from build123d import *

# Parameters (mm, degrees)
BOSS_EXTRUDE1_DEPTH = 120
SKETCH3_W           = 42
SKETCH3_H           = 12
CUT_EXTRUDE2_DEPTH  = 30
SKETCH6_R           = 2.5
CUT_EXTRUDE3_DEPTH  = 30
SKETCH8_W           = 42.8
SKETCH8_H           = 12.8
BOSS_EXTRUDE2_DEPTH = 30
SKETCH9_R           = 2.5
CUT_EXTRUDE4_DEPTH  = 30


with BuildPart() as part:
    # Sketch1 → Boss-Extrude1 (new body)
    with BuildSketch(Plane(origin=(0, 0, 0), x_dir=(1, 0, 0), z_dir=(0, 1, 0))):
        with BuildLine():
            Line((2, 0), (48, 0))
            ThreePointArc((48, 0), (49.414213562, 0.585786438), (50, 2))
            Line((50, 2), (50, 18))
            ThreePointArc((50, 18), (49.414213562, 19.414213562), (48, 20))
            Line((48, 20), (2, 20))
            ThreePointArc((2, 20), (0.585786438, 19.414213562), (0, 18))
            Line((0, 18), (0, 2))
            ThreePointArc((0, 2), (0.585786438, 0.585786438), (2, 0))
        make_face()
    extrude(amount=BOSS_EXTRUDE1_DEPTH)

    # Sketch3 → Cut-Extrude2 (cut)
    with BuildSketch(Plane.XZ):
        with Locations((25, -10)):
            Rectangle(SKETCH3_W, SKETCH3_H)
    extrude(amount=-CUT_EXTRUDE2_DEPTH, mode=Mode.SUBTRACT)

    # Sketch6 → Cut-Extrude3 (cut)
    with BuildSketch(Plane.XY):
        with Locations((25, 105)):
            Circle(SKETCH6_R)
        with Locations((25, 15)):
            Circle(SKETCH6_R)
    extrude(amount=-CUT_EXTRUDE3_DEPTH, mode=Mode.SUBTRACT)

    # Sketch8 → Boss-Extrude2 (add)
    with BuildSketch(Plane(origin=(0, 120, 0), x_dir=(1, 0, 0), z_dir=(0, 1, 0))):
        with Locations((25, 10)):
            Rectangle(SKETCH8_W, SKETCH8_H)
    extrude(amount=BOSS_EXTRUDE2_DEPTH)

    # Sketch9 → Cut-Extrude4 (cut)
    with BuildSketch(Plane.XY.offset(-3.6)):
        with Locations((25, 135)):
            Circle(SKETCH9_R)
    extrude(amount=-CUT_EXTRUDE4_DEPTH, mode=Mode.SUBTRACT)


solid = part.part
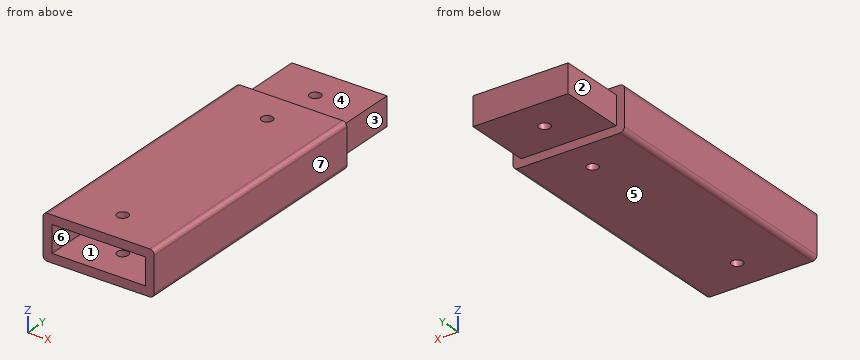
Build history of the part. All positions in model axes, mm. Face numbers are marked on the shaded views. A direction names the side the tool comes from. Round coordinates to 2 decimals unless told otherwise and drop trailing zeros. Loops run counter-clockwise (first coordinate to the right, second up) from the corner with the lowest first, then second, coordinate; pieces in that order, holes last. Notation, with made-up numbers: (-10.75, 85) -> (37.25, 85) arc R25 ccw to (37.25, 116) -> close; hole circle Ø11 at (-23.75, 72.5). An arc over 180 degrees is marked (long way). Answer in a Markdown table with one row per item.
Item 1: Drill centre lines: L1, parallel to Y at x = 25, z = -9.5; L2, parallel to Y at x = 25, z = -0.85; L3, parallel to Z at x = 21, y = 23. Where is each one in solid material? Low to high. Write a range as [from, to].
Answers below:
| item | result |
|---|---|
| L1 | y = [30, 102.5], [107.5, 132.5], [137.5, 150] |
| L2 | y = [0, 12.5], [17.5, 102.5], [107.5, 120] |
| L3 | z = [-20, -16], [-4, 0] |
Item 2: Saw through at D-D (x = 19). Write the cut outline in (y, z), and give its area (3 significant figures).
Answers below:
| item | result |
|---|---|
| outline | (0, -20) -> (120, -20) -> (120, -16.4) -> (150, -16.4) -> (150, -3.6) -> (120, -3.6) -> (120, 0) -> (0, 0) -> (0, -4) -> (30, -4) -> (30, -16) -> (0, -16) -> close |
| area | 2,420 mm² |
Item 3: Saw through at C-C (z = -12.75). Write the cut outline in (x, y).
Answers below:
| item | result |
|---|---|
| outline | (0, 0) -> (4, 0) -> (4, 30) -> (46, 30) -> (46, 0) -> (50, 0) -> (50, 120) -> (46.4, 120) -> (46.4, 150) -> (3.6, 150) -> (3.6, 120) -> (0, 120) -> close; hole circle Ø5 at (25, 105); hole circle Ø5 at (25, 135) |
Item 4: Saw through at A-A (x = 25). Write the cut outline in (y, z), and give its area (3 significant figures).
Answers below:
| item | result |
|---|---|
| outline | (0, -20) -> (12.5, -20) -> (12.5, -16) -> (0, -16) -> close; (0, -4) -> (12.5, -4) -> (12.5, 0) -> (0, 0) -> close; (17.5, -20) -> (102.5, -20) -> (102.5, 0) -> (17.5, 0) -> (17.5, -4) -> (30, -4) -> (30, -16) -> (17.5, -16) -> close; (107.5, -20) -> (120, -20) -> (120, -16.4) -> (132.5, -16.4) -> (132.5, -3.6) -> (120, -3.6) -> (120, 0) -> (107.5, 0) -> close; (137.5, -16.4) -> (150, -16.4) -> (150, -3.6) -> (137.5, -3.6) -> close |
| area | 2,220 mm² |
Item 5: Pin check, flat tips, straight feed: pin 1 (15 mm diameter, centred on x = 28, y = 131.5, fed in from -Z); pin 2 (1.5 mm diameter, centred on x = 10, z = -18, fed in from +Y); pin 3 (4 mm diameter, centred on y = 131.5, z = -12.5, fed in from -X). Stop position of each tip, or through.
Answers below:
| item | result |
|---|---|
| pin 1 | stops at z = -16.4 |
| pin 2 | stops at y = 120 |
| pin 3 | stops at x = 3.6 |
Item 6: Saw through at B-B (y = 15). Write the cut outline in (x, z), and give its area (3 significant figures).
Answers below:
| item | result |
|---|---|
| outline | (0, -18) arc R2 ccw to (2, -20) -> (22.5, -20) -> (22.5, -16) -> (4, -16) -> (4, -4) -> (22.5, -4) -> (22.5, 0) -> (2, 0) arc R2 ccw to (0, -2) -> close; (27.5, -20) -> (48, -20) arc R2 ccw to (50, -18) -> (50, -2) arc R2 ccw to (48, 0) -> (27.5, 0) -> (27.5, -4) -> (46, -4) -> (46, -16) -> (27.5, -16) -> close |
| area | 453 mm² |
Item 7: Which spindle directions (+Z, -Z, +X, -X, +Y, -Y) get a long thin tool onto all of the face, cutting with end or side? Do the marked faces 1, 2, 3 and 4. Say none if no direction does.
Answers below:
| item | result |
|---|---|
| face 1 | -Y |
| face 2 | +Z, -Z, -X, +Y |
| face 3 | +Z, -Z, +X, +Y |
| face 4 | +Z, +X, -X, +Y |
Item 8: Mould opens along X. For the marked faces 5, 6 and 7 say: +X half, -X half, draft (parallel to the pull), parting line (faces both ways), or undercut.
Answers below:
| item | result |
|---|---|
| face 5 | draft |
| face 6 | undercut |
| face 7 | +X half |
